Geometry: final body of the model. Coordinates: model frame, mm. A direction names the side the tool comes from. Give positions to 0.01 mm unless a question says otherwise; leave off trailing zeros. Order: outer loops, then holes, each group sorted by start corner. A loop starts at its lowest first (then second) coordinate and runs counter-clockwise, first axis right, second up. Notation, with made-up numbers: (34.25, 35.5) -> (76.25, 35.5) arc R22 cw to (76.25, 65.5) -> close; hole circle Ø6 at (35, 85.25). An arc over 180 degrees is marked (long way). Answer in a Markdown table with one row per item. Add a question column.
Q1. Line query: line 1 along Y through (x, z) = (0, 2.05); line 2 along Y through (x, z) = (0, 8.25); line 3 along X through (y, z) = (0, 9.8). Output: solid intervals per line, ascending. Write a range as from..to.
Q2. Set-up query: faces 4 (the face through (-33, 2, 9.1)), 5 (the face through (1, 1, 10)), 6 (the face through (-0.716, 33.737, 7.831)). Return all of +Z, -Z, +X, -X, +Y, -Y with unobstructed straight access to the full face (end or side cutting, diameter ignored); none if empty.
Q3. Cut plane C-C on x = -34.35. Return the cut outline in (y, z).
Q4. Contact query for flat-ended pins moving along their axis: P1, Ø9, axis at x = 34.35, y = 0, coming from the +Z side; P2, Ø2, axis at x = -24.5, z = 5.5, coming from the -Y side; P3, Ø5.5, axis at x = -2, y = 28.5, coming from the +Z side; P4, Ø1.7, axis at x = 35.5, y = 1, coming from the -Z side. Output: stop coordinate, or through.
Q5. Pull-direction query (X, two-part tool) for faces 1 (the face through (-4.054, -24.567, 7.831)), 2 (the face through (-21, 21, 5)), 3 (the face through (39.93, 0.05, 5.07)); classes: +X half, -X half, draft (parallel to the pull), parting line (faces both ways), or undercut.
Q6. Cut plane A-A on x = 0. Return the cut outline in (y, z), and give its area (3 significant figures).
Q7. Cut plane D-D on z = 6.75. Return the cut outline in (x, y).
Q8. Cut plane B-B on y = 0. Return the cut outline in (x, z).
from build123d import *

# Parameters (mm, degrees)
SKETCH1_R                                           = 2.25
BOSS_EXTRUDE1_DEPTH                                 = 10
SKETCH2_R                                           = 2.8
CUT_EXTRUDE1_DEPTH                                  = 9.1
CBORE_FOR_M6_HEX_SOCKET_HEAD_CAP_SCREW1_D           = 6.6
CBORE_FOR_M6_HEX_SOCKET_HEAD_CAP_SCREW1_CBORE_D     = 11
CBORE_FOR_M6_HEX_SOCKET_HEAD_CAP_SCREW1_CBORE_DEPTH = 4.4
CBORE_FOR_M6_HEX_SOCKET_HEAD_CAP_SCR_2_D            = 6.6
CBORE_FOR_M6_HEX_SOCKET_HEAD_CAP_SCR_2_CBORE_D      = 11
CBORE_FOR_M6_HEX_SOCKET_HEAD_CAP_SCR_2_CBORE_DEPTH  = 4.4
FILLET2_R                                           = 5


with BuildPart() as part:
    # Sketch1 → Boss-Extrude1 (new body)
    with BuildSketch(Plane.XY):
        Polygon((-42, 0), (0, 42), (42, 0), (0, -42), align=None)
        with Locations((-34.35, 0)):
            Circle(SKETCH1_R, mode=Mode.SUBTRACT)
        with Locations((34.35, 0)):
            Circle(SKETCH1_R, mode=Mode.SUBTRACT)
    extrude(amount=BOSS_EXTRUDE1_DEPTH)

    # Sketch2 → Cut-Extrude1 (cut)
    with BuildSketch(Plane.XY):
        with Locations((34.35, 0)):
            Circle(SKETCH2_R)
        with Locations((-34.35, 0)):
            Circle(SKETCH2_R)
    extrude(amount=CUT_EXTRUDE1_DEPTH, mode=Mode.SUBTRACT)

    # CBORE for M6 Hex Socket Head Cap Screw1 (through all)
    with Locations(Plane(origin=(0, 28.284271247, 10), x_dir=(1, 0, 0), z_dir=(0, 0, 1))):
        with Locations((0, 0), (0, -56.568542494)):
            CounterBoreHole(CBORE_FOR_M6_HEX_SOCKET_HEAD_CAP_SCREW1_D / 2, CBORE_FOR_M6_HEX_SOCKET_HEAD_CAP_SCREW1_CBORE_D / 2, CBORE_FOR_M6_HEX_SOCKET_HEAD_CAP_SCREW1_CBORE_DEPTH)

    # CBORE for M6 Hex Socket Head Cap Scr 2 (through all)
    with Locations(Plane(origin=(55.283571739, 20.980488531, 0), x_dir=(1, 0, 0), z_dir=(0, 0, 1))):
        with Locations((0, 0)):
            CounterBoreHole(CBORE_FOR_M6_HEX_SOCKET_HEAD_CAP_SCR_2_D / 2, CBORE_FOR_M6_HEX_SOCKET_HEAD_CAP_SCR_2_CBORE_D / 2, CBORE_FOR_M6_HEX_SOCKET_HEAD_CAP_SCR_2_CBORE_DEPTH)

    # Fillet2
    fillet2_edges = [part.edges().sort_by_distance(p)[0] for p in [
        (-42, 0, 5),
        (0, 42, 5),
        (42, 0, 5),
        (0, -42, 5),
    ]]
    fillet(fillet2_edges, radius=FILLET2_R)


solid = part.part
Completed:
| question | item | result |
|---|---|---|
| 1 | line 1 | y = -39.93..-31.58, -24.98..24.98, 31.58..39.93 |
| 1 | line 2 | y = -39.93..-33.78, -22.78..22.78, 33.78..39.93 |
| 1 | line 3 | x = -39.93..-36.6, -32.1..32.1, 36.6..39.93 |
| 2 | face 4 | -Z |
| 2 | face 5 | +Z, +X, -X, +Y, -Y |
| 2 | face 6 | +Z |
| 3 | outline | (-7.65, 0) -> (-2.8, 0) -> (-2.8, 9.1) -> (-2.25, 9.1) -> (-2.25, 10) -> (-7.65, 10) -> close; (2.25, 9.1) -> (2.8, 9.1) -> (2.8, 0) -> (7.65, 0) -> (7.65, 10) -> (2.25, 10) -> close |
| 4 | P1 | stops at z = 10 |
| 4 | P2 | stops at y = -18.5 |
| 4 | P3 | stops at z = 5.6 |
| 4 | P4 | stops at z = 9.1 |
| 5 | face 1 | undercut |
| 5 | face 2 | -X half |
| 5 | face 3 | +X half |
| 6 | outline | (-39.93, 0) -> (-31.58, 0) -> (-31.58, 5.6) -> (-33.78, 5.6) -> (-33.78, 10) -> (-39.93, 10) -> close; (-24.98, 0) -> (24.98, 0) -> (24.98, 5.6) -> (22.78, 5.6) -> (22.78, 10) -> (-22.78, 10) -> (-22.78, 5.6) -> (-24.98, 5.6) -> close; (31.58, 0) -> (39.93, 0) -> (39.93, 10) -> (33.78, 10) -> (33.78, 5.6) -> (31.58, 5.6) -> close |
| 6 | area | 628 mm² |
| 7 | outline | (-38.46, -3.54) -> (-3.54, -38.46) arc R5 ccw to (3.54, -38.46) -> (38.46, -3.54) arc R5 ccw to (38.46, 3.54) -> (3.54, 38.46) arc R5 ccw to (-3.54, 38.46) -> (-38.46, 3.54) arc R5 ccw to start; hole circle Ø5.6 at (-34.35, 0); hole circle Ø11 at (0, -28.28); hole circle Ø11 at (0, 28.28); hole circle Ø5.6 at (34.35, 0) |
| 8 | outline | (-39.93, 0) -> (-37.15, 0) -> (-37.15, 9.1) -> (-36.6, 9.1) -> (-36.6, 10) -> (-39.93, 10) -> close; (-32.1, 9.1) -> (-31.55, 9.1) -> (-31.55, 0) -> (31.55, 0) -> (31.55, 9.1) -> (32.1, 9.1) -> (32.1, 10) -> (-32.1, 10) -> close; (36.6, 9.1) -> (37.15, 9.1) -> (37.15, 0) -> (39.93, 0) -> (39.93, 10) -> (36.6, 10) -> close |
